```python
from build123d import *

# Parameters (mm, degrees)
CUT_EXTRUDE_1_DEPTH = 21.223748416
CUT_EXTRUDE_2_REACH = 20.762
SKETCH_3_R          = 1.5
SKETCH_5_R          = 1.7
CUT_EXTRUDE_3_DEPTH = 21.223748416
SKETCH_6_R          = 4
CUT_EXTRUDE_4_DEPTH = 19.761663039


with BuildPart() as part:
    # 草图1 → 旋转1 (revolve)
    with BuildSketch(Plane(origin=(0, 0, 0), x_dir=(1, 0, 0), z_dir=(0, 1, 0))):
        Polygon((0, 0), (0, 12), (3, 12), (3, 7), (11, 7), (11, 4), (3, 4), (3, 0), align=None)
    revolve(axis=Axis((3, 0, 0), (-1, 0, 0)))

    # 草图2 → 切除-拉伸1 (cut, through all)
    with BuildSketch(Plane(origin=(11, 0, 0), x_dir=(0, 0, -1), z_dir=(1, 0, 0))):
        with BuildLine():
            Line((1.5, -5.4), (1.5, -3.708099244))
            ThreePointArc((1.5, -3.708099244), (0, -4), (-1.5, -3.708099244))
            Line((-1.5, -3.708099244), (-1.5, -5.4))
            Line((-1.5, -5.4), (1.5, -5.4))
        make_face()
        with BuildLine():
            Line((-1.5, 5.4), (1.5, 5.4))
            Line((1.5, 5.4), (1.5, 3.708099244))
            ThreePointArc((1.5, 3.708099244), (0, 4), (-1.5, 3.708099244))
            Line((-1.5, 3.708099244), (-1.5, 5.4))
        make_face()
    extrude(amount=-CUT_EXTRUDE_1_DEPTH, mode=Mode.SUBTRACT)

    # 草图3 → 切除-拉伸2 (cut, up to next)
    with BuildSketch(Plane(origin=(3, 0, 0), x_dir=(0, 0, -1), z_dir=(1, 0, 0)), mode=Mode.PRIVATE) as cut_extrude_2_sk1:
        with Locations((0, 9)):
            Circle(SKETCH_3_R)
    cut_extrude_2_tool1 = extrude(cut_extrude_2_sk1.sketch, amount=-CUT_EXTRUDE_2_REACH, mode=Mode.PRIVATE) & part.part
    # 草图3 → 切除-拉伸2 (cut, up to next)
    with BuildSketch(Plane(origin=(3, 0, 0), x_dir=(0, 0, -1), z_dir=(1, 0, 0)), mode=Mode.PRIVATE) as cut_extrude_2_sk2:
        with Locations((9, 0)):
            Circle(SKETCH_3_R)
    cut_extrude_2_tool2 = extrude(cut_extrude_2_sk2.sketch, amount=-CUT_EXTRUDE_2_REACH, mode=Mode.PRIVATE) & part.part
    # 草图3 → 切除-拉伸2 (cut, up to next)
    with BuildSketch(Plane(origin=(3, 0, 0), x_dir=(0, 0, -1), z_dir=(1, 0, 0)), mode=Mode.PRIVATE) as cut_extrude_2_sk3:
        with Locations((0, -9)):
            Circle(SKETCH_3_R)
    cut_extrude_2_tool3 = extrude(cut_extrude_2_sk3.sketch, amount=-CUT_EXTRUDE_2_REACH, mode=Mode.PRIVATE) & part.part
    # 草图3 → 切除-拉伸2 (cut, up to next)
    with BuildSketch(Plane(origin=(3, 0, 0), x_dir=(0, 0, -1), z_dir=(1, 0, 0)), mode=Mode.PRIVATE) as cut_extrude_2_sk4:
        with Locations((-9, 0)):
            Circle(SKETCH_3_R)
    cut_extrude_2_tool4 = extrude(cut_extrude_2_sk4.sketch, amount=-CUT_EXTRUDE_2_REACH, mode=Mode.PRIVATE) & part.part
    add(cut_extrude_2_tool1.solids().sort_by_distance((3, 9, 0))[0], mode=Mode.SUBTRACT)
    add(cut_extrude_2_tool2.solids().sort_by_distance((3, 0, -9))[0], mode=Mode.SUBTRACT)
    add(cut_extrude_2_tool3.solids().sort_by_distance((3, -9, 0))[0], mode=Mode.SUBTRACT)
    add(cut_extrude_2_tool4.solids().sort_by_distance((3, 0, 9))[0], mode=Mode.SUBTRACT)

    # 草图5 → 切除-拉伸3 (cut, through all)
    with BuildSketch(Plane.ZY):
        Circle(SKETCH_5_R)
    extrude(amount=-CUT_EXTRUDE_3_DEPTH, mode=Mode.SUBTRACT)

    # 草图6 → 切除-拉伸4 (cut, through all)
    with BuildSketch(Plane(origin=(3, 0, 0), x_dir=(0, 0, -1), z_dir=(1, 0, 0))):
        Circle(SKETCH_6_R)
    extrude(amount=-CUT_EXTRUDE_4_DEPTH, mode=Mode.SUBTRACT)


solid = part.part
```
Verification items for the finished model (mm, model axes). A direction names the side the tool comes from. Round coordinates to 2 decimals unless told otherwise and drop trailing zeros. Order: outer loops, then holes, each group sorted by start corner. A loop starts at its lowest first (then second) coordinate and runs counter-clockwise, first axis right, second up. Notation, with made-up numbers: (47.25, 68.5) - (65.25, 68.5) arc R13 ccw to (65.25, 90.5) - close; hole circle Ø8 at (27.5, -37). An arc over 180 degrees is marked (long way). Use CSV: the item, a comma, the result in double quotes.
(1) Thickness scan on probe 1 along Y at (x, z) = (1.35, 0); probe 2 along Z at (x, y) = (2.75, 1.25); probe 3 along Y at (x, z) = (9.5, -0.25). Record the ranges inside material, lowest first. Write a range as from..to.
Entries:
probe 1,"-12..-10.5, -7.5..-5.4, 5.4..7.5, 10.5..12"
probe 2,"-11.93..-9.83, -8.17..-3.8, 3.8..8.17, 9.83..11.93"
probe 3,"-7..-5.4, 5.4..7"
(2) Gauge pin test, flat ends, axial feed: pin 1 Ø0.9 at (x, z) = (4, -0.5) entering from -Y; pin 2 Ø1.9 at (x, y) = (6, 4.5) entering from +Z; pin 3 Ø1.4 at (x, y) = (8, -4.5) entering from +Z. Record the tip position at first contact, or that the pin passes through.
Entries:
pin 1,"y = -7"
pin 2,"z = 6.03"
pin 3,"z = 5.88"
(3) Section check C-C on y = 0. Record the boundary of the cut face in (x, z), and give its area (3 significant figures).
Entries:
outline,"(0, -12) - (3, -12) - (3, -10.5) - (0, -10.5) - close; (0, -7.5) - (3, -7.5) - (3, -7) - (11, -7) - (11, -4) - (0, -4) - close; (0, 4) - (11, 4) - (11, 7) - (3, 7) - (3, 7.5) - (0, 7.5) - close; (0, 10.5) - (3, 10.5) - (3, 12) - (0, 12) - close"
area,"78.0 mm^2"
(4) Section check A-A on z = 0. Record the boundary of the cut face in (x, y).
Entries:
outline,"(0, -12) - (3, -12) - (3, -10.5) - (0, -10.5) - close; (0, -7.5) - (3, -7.5) - (3, -7) - (11, -7) - (11, -5.4) - (0, -5.4) - close; (0, 5.4) - (11, 5.4) - (11, 7) - (3, 7) - (3, 7.5) - (0, 7.5) - close; (0, 10.5) - (3, 10.5) - (3, 12) - (0, 12) - close"
(5) Access from +Z, -Z, +X, -X, +Y, -Y to the whole of each face (thin tool, end or side, straight path). Record for faces 1 (the face through (6, 0, -4)), 2 (the face through (7.056, 2.681, -6.466)), 3 (the face through (11, 3, -3)).
Entries:
face 1,"+X, -X"
face 2,"+X"
face 3,"+Z, -Z, +X, +Y, -Y"
(6) Section check D-D on z = 9. Record the boundary of the cut face in (x, y), and give its area (3 significant figures).
Entries:
outline,"(0, -7.94) - (3, -7.94) - (3, -1.5) - (0, -1.5) - close; (0, 1.5) - (3, 1.5) - (3, 7.94) - (0, 7.94) - close"
area,"38.6 mm^2"
(7) Mould release check, pull along Z, two halves, no side actions. Record for faces 4 (the face through (0, -3, -3)), 5 (the face through (1.52, -0.53, 11.99)), 6 (the face through (6, 5, 1.5)): released by +Z, released by -Z, zero draft, split by the parting line, or undercut.
Entries:
face 4,"zero draft"
face 5,"split by the parting line"
face 6,"undercut"
(8) Section check B-B on x = 9.5. Record the boundary of the cut face in (y, z).
Entries:
outline,"circle Ø14 at (0, 0); hole (-5.4, -1.5) - (-3.71, -1.5) arc R4 ccw to (3.71, -1.5) - (5.4, -1.5) - (5.4, 1.5) - (3.71, 1.5) arc R4 ccw to (-3.71, 1.5) - (-5.4, 1.5) - close"
